Source: CAD feature listing. Evaluate the final solid. Frame: model axes, mm. Face numbers are marked on the shaded views. A direction names the side the tool comes from. Round coordinates to 2 decimals unless told otherwise and drop trailing zeros. Order: outer loops, then holes, each group sorted by start corner. A loop starts at its lowest first (then second) coordinate and runs counter-clockwise, first axis right, second up. Notation, with made-up numbers: M -29.5,83 L -1.5,83 A19 ccw -1.5,94 Z; hole C -1,-25.75 d2. An arc over 180 degrees is marked long. Use one line per item in the form item = value. Start each with the question number.
Q1. Section C-C (x = -5). Return the cut outline in (y, z).
Q2. Material intervals for probe 1 along Z at (x, y) = (0, -4); probe 2 along X at (y, z) = (3, 5.25); probe 3 along X at (y, z) = (-15, 6.5), sorted ascending.
Q3. Section D-D (y = -8). Return the cut outline in (x, z).
Q4. Section B-B (y = 16). Return the cut outline in (x, z), plus the area to 3 significant figures.
Q5. Reachability of the marked faces 5 and 6 from +Z, -Z, +X, -X, +Y, -Y: full face, straight path, thin tool, end or side. Return the list, or none.
Q6. Pull-direction query (X, two-part tool) for the marked faces 1, 2, 3 and 4; classes: pulls with the +X half, pulls with the -X half, needs draft (parallel to the pull), parting line crosses it, or undercut.
Q7. Section A-A (z = 6.5). Return the cut outline in (x, y), plus the area to 3 significant figures.
Q8. Contact query for flat-ended pins moving along their axis: pin 1 (5 mm diameter, centred on x = 30.5, y = -2.5, fed in from -Z); pin 2 (3 mm diameter, centred on y = -18, z = 7, fed in from +X); pin 3 (1.5 mm diameter, centred on y = 6.5, z = 8, fed in from +X); pin 4 (6.5 mm diameter, centred on x = -6, y = -7, fed in from +Z). Output: stop coordinate, or through.
from build123d import *

# Parameters (mm, degrees)
F1_DEPTH = 10
F2_R     = 11
F3_DEPTH = 5


# Not quite as in the source:
# - a feature names something its author has since deleted; it is built from what else it names


with BuildPart() as f1:
    # F0 (on Top) → F1 (new body)
    with BuildSketch(Plane.XY):
        Polygon((-25, -25), (25, -25), (25, -10.8146222424), (25, -10.5146222424), (15, -7.2654252801), (15, 7.2654252801), (25, 10.5146222424), (25, 10.8146222424), (25, 25), (11.5660844666, 25), (12.9312755504, 20.7983738762), (0, 11.4032522475), (-12.9312755504, 20.7983738762), (-11.5660844666, 25), (-25, 25), align=None)
        Polygon((25, 10.5146222424), (25, -10.5146222424), (28.8196601125, -11.7557050458), (37.360679775, 0), (28.8196601125, 11.7557050458), align=None)
        Polygon((15, -7.2654252801), (25, -10.5146222424), (25, 10.5146222424), (15, 7.2654252801), align=None)
        Polygon((25, 10.8146222424), (25, 10.5146222424), (28.8196601125, 11.7557050458), (37.360679775, 0), (37.760679775, 0), (28.8196601125, 12.0557050458), align=None)
        Polygon((25, -10.5146222424), (25, -10.8146222424), (28.8196601125, -12.0557050458), (29.200082719, -12.1793118436), (37.760679775, 0), (37.360679775, 0), (28.8196601125, -11.7557050458), align=None)
    extrude(amount=F1_DEPTH)

    # F2 (on face) → F3 (cut)
    with BuildSketch(Plane.XY.offset(10)):
        with Locations((-6.0343622248, -6.7983738762)):
            Circle(F2_R)
    extrude(amount=-F3_DEPTH, mode=Mode.SUBTRACT)


solid = f1.part
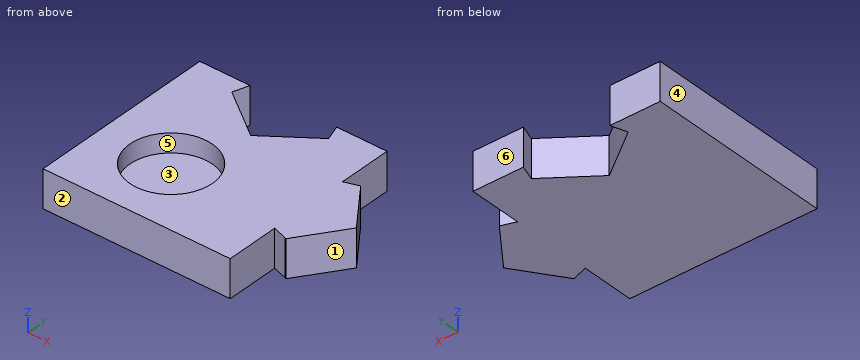
Results list:
q1.outline = M -25,0 L 15.04,0 L 15.04,10 L 4.15,10 L 4.15,5 L -17.75,5 L -17.75,10 L -25,10 Z
q2.probe_1 = 0 to 5
q2.probe_2 = -25 to -11.03, -1.04 to 35.54
q2.probe_3 = -25 to -13.36, 1.3 to 25
q3.outline = M -25,0 L 32.14,0 L 32.14,10 L 4.9,10 L 4.9,5 L -16.97,5 L -16.97,10 L -25,10 Z
q4.outline = M -25,0 L -6.33,0 L -6.33,10 L -25,10 Z; M 6.33,0 L 25,0 L 25,10 L 6.33,10 Z
q4.area = 373 mm2
q5.face_5 = +Z
q5.face_6 = +Z, -Z, +X, -X, +Y
q6.face_1 = pulls with the +X half
q6.face_2 = needs draft
q6.face_3 = undercut
q6.face_4 = pulls with the -X half
q7.outline = M -25,-25 L 25,-25 L 25,-10.81 L 29.2,-12.18 L 37.76,0 L 28.82,12.06 L 25,10.81 L 25,25 L 11.57,25 L 12.93,20.8 L 0,11.4 L -12.93,20.8 L -11.57,25 L -25,25 Z; hole C -6.03,-6.8 d22
q7.area = 2,090 mm2
q8.pin_1 = 0
q8.pin_2 = 25
q8.pin_3 = 33.5
q8.pin_4 = 5
